Verification items for the finished model (mm, model axes). Face numbers are marked on the shaded views. Give positions to 0.01 mm unless a question says otherwise; leave off trailing zeros. Write each loop counter-clockwise with the first axis right and the second up, starting at its lowest first coordinate (ties: lowest second). Pieces come first, ordered by that corner, then holes. Notation, with made-up numbers: (22.5, 37) -> (35.5, 37) arc R32 ccw to (35.5, 74) -> close; hole circle Ø2 at (3, 82). An arc over 180 degrees is marked (long way). Write item = value, one per line.
from build123d import *

# Parameters (mm, degrees)
SKETCH1_R           = 50
BOSS_EXTRUDE1_DEPTH = 20
SKETCH2_R           = 2.5
CUT_EXTRUDE1_DEPTH  = 74.484692283


with BuildPart() as part:
    # Sketch1 → Boss-Extrude1 (new body)
    with BuildSketch(Plane.XY):
        Circle(SKETCH1_R)
        with BuildLine():
            Line((-2, 13.856406461), (-2, 15))
            Line((-2, 15), (2, 15))
            Line((2, 15), (2, 13.856406461))
            ThreePointArc((2, 13.856406461), (0, -14), (-2, 13.856406461))
        make_face(mode=Mode.SUBTRACT)
    extrude(amount=BOSS_EXTRUDE1_DEPTH)

    # Sketch2 → Cut-Extrude1 (cut, through all)
    with BuildSketch(Plane.XY.offset(20)):
        with Locations((0, -30)):
            Circle(SKETCH2_R)
        with Locations((-25.980762114, -15)):
            Circle(SKETCH2_R)
        with Locations((-25.980762114, 15)):
            Circle(SKETCH2_R)
        with Locations((0, 30)):
            Circle(SKETCH2_R)
        with Locations((25.980762114, 15)):
            Circle(SKETCH2_R)
        with Locations((25.980762114, -15)):
            Circle(SKETCH2_R)
    extrude(amount=-CUT_EXTRUDE1_DEPTH, mode=Mode.SUBTRACT)


solid = part.part
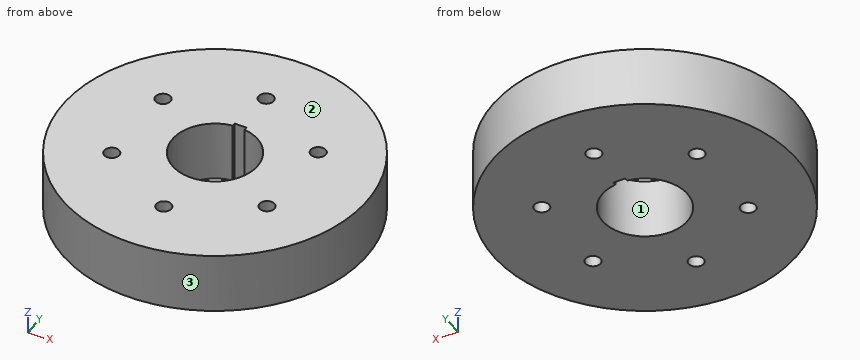
Item 1: Sectioned sample at B-B on z = 17.5. Record the cut outline in (x, y), then the cut area to 3 significant figures.
Response values:
outline = circle Ø100 at (0, 0); hole circle Ø5 at (-25.98, -15); hole circle Ø5 at (-25.98, 15); hole circle Ø5 at (0, -30); hole circle Ø5 at (0, 30); hole (-2, 13.86) arc R14 ccw (long way) to (2, 13.86) -> (2, 15) -> (-2, 15) -> close; hole circle Ø5 at (25.98, -15); hole circle Ø5 at (25.98, 15)
area = 7,120 mm^2
Item 2: Sectioned sample at C-C on x = 0. Record the cut outline in (y, z), then the cut area to 3 significant figures.
Response values:
outline = (-50, 0) -> (-32.5, 0) -> (-32.5, 20) -> (-50, 20) -> close; (-27.5, 0) -> (-14, 0) -> (-14, 20) -> (-27.5, 20) -> close; (15, 0) -> (27.5, 0) -> (27.5, 20) -> (15, 20) -> close; (32.5, 0) -> (50, 0) -> (50, 20) -> (32.5, 20) -> close
area = 1,220 mm^2
Item 3: Material ranges on line 1 (Y direction, x = 0, z = 8.25); line 2 (X direction, y = 16.5, z = 7.5); line 3 (X direction, y = -17, z = 10.25), recorded low to high.
Response values:
line_1 = -50 to -32.5, -27.5 to -14, 15 to 27.5, 32.5 to 50
line_2 = -47.2 to -27.98, -23.98 to 23.98, 27.98 to 47.2
line_3 = -47.02 to -27.48, -24.48 to 24.48, 27.48 to 47.02
Item 4: Sectioned sample at D-D on y = 30. Record the cut outline in (x, z).
Response values:
outline = (-40, 0) -> (-2.5, 0) -> (-2.5, 20) -> (-40, 20) -> close; (2.5, 0) -> (40, 0) -> (40, 20) -> (2.5, 20) -> close
Item 5: Mould release check, pull along Y, two halves, no side actions. Record for the marked faces 1, 2 and 3: +Y half, -Y half, draft (parallel to the pull), parting line (faces both ways), or undercut.
Response values:
face_1 = undercut
face_2 = draft
face_3 = parting line
Item 6: Go/stop test with flat-tipped pins: P1, Ø2, axis at x = -33, z = 15, coming from the -Y side; P2, Ø10, axis at y = -9, z = 6.5, coming from the -X side; P3, Ø1.2, axis at x = -0.5, z = 15, coming from the -Y side. Record where each tip stops, or that it passes through.
Response values:
P1 = -38.42
P2 = -49.84
P3 = -50
Item 7: Sectioned sample at A-A on y = 0. Record the cut outline in (x, z).
Response values:
outline = (-50, 0) -> (-14, 0) -> (-14, 20) -> (-50, 20) -> close; (14, 0) -> (50, 0) -> (50, 20) -> (14, 20) -> close
